Can you work these out from the model? Positions are in its coordinate system, mm. Face numbers are marked on the shaded views. Coordinates: 2 decimals unless noted, no trailing zeros. Order: outer loops, then holes, each group sorted by start corner. A loop starts at its lowest first (then second) coordinate and runs counter-clockwise, first axis right, second up. Notation, with made-up numbers: (34.5, -24) - (52.5, -24) arc R27 ccw to (52.5, -4) - close; hole circle Ø10 at (67.5, 54). An arc over 180 degrees is marked (long way). Use a Markdown table: item, result. Add a question column.
(1) I want a section at B-B (y = 2.05). List the corners of the cut face in (x, z) for me.
(2) I want a section at C-C (z = -0.5). List the corners of the cut face in (x, y) for me.
(3) If I drill on L1, parallel to Z at x = 22.25, y = 1.3; L2, parallel to Y at x = 6, z = 0.25; L3, parallel to Y at x = 10, z = 1, over which ranges is the centre line in solid material (lowest first)? Write a range as [from, to].
(4) I want a section at A-A (z = 2). List the corners of the cut face in (x, y) for me, and give its area (3 significant figures).
(5) We'd pull the mould along Z, two halves only. Please class the marked faces 1, 2 and 3: pulls with the +Z half, pulls with the -Z half, needs draft (parallel to the pull), parting line crosses it, or undercut.
(6) I want a section at D-D (z = 5.75). List the corners of the cut face in (x, y) for me, and give its area (3 significant figures).
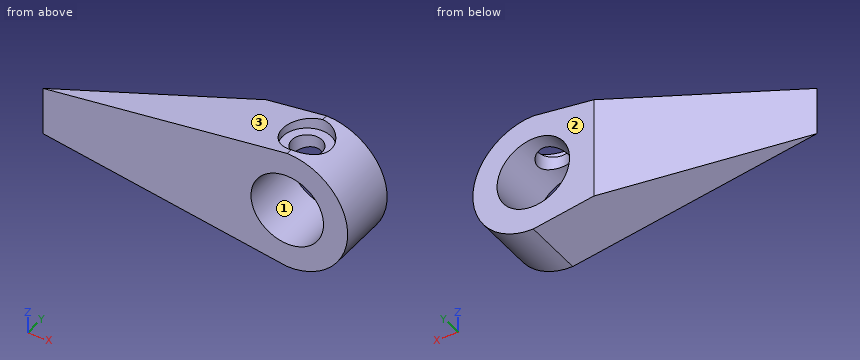
```python
from build123d import *

# Parameters (mm, degrees)
BOSS_EXTRUDE4_DEPTH     = 4
BOSS_EXTRUDE6_DEPTH     = 5
CUT_EXTRUDE3_REACH      = 28.627
CUT_EXTRUDE2_REACH      = 28.627
SKETCH9_R               = 3
CUT_EXTRUDE4_REACH      = 29.568
CUT_EXTRUDE4_END_RADIUS = 3
SKETCH12_R              = 1.25
SKETCH13_R              = 2
CUT_EXTRUDE5_DEPTH      = 1


with BuildPart() as part:
    # Sketch1 → Boss-Extrude4 (new body)
    with BuildSketch(Plane.XY):
        Polygon((0, 0), (15.198684154, 5), (15.198684154, 0), align=None)
    extrude(amount=BOSS_EXTRUDE4_DEPTH)

    # Sketch7 → Boss-Extrude6 (add)
    with BuildSketch(Plane(origin=(0, 0, 0), x_dir=(1, 0, 0), z_dir=(0, 1, 0))):
        with BuildLine():
            Line((20.198684154, 3), (0, 0))
            Line((0, 0), (15.198684154, 0))
            Line((15.198684154, 0), (15.198684154, -4))
            Line((15.198684154, -4), (0, -4))
            Line((0, -4), (20.198684154, -7))
            ThreePointArc((20.198684154, -7), (25.198684154, -2), (20.198684154, 3))
        make_face()
    extrude(amount=BOSS_EXTRUDE6_DEPTH)

    # Sketch10 → Cut-Extrude3 (cut, up to next)
    with BuildSketch(Plane.XY, mode=Mode.PRIVATE) as cut_extrude3_sk1:
        Polygon((0, 0), (0, 5), (15.198684154, 5), align=None)
    cut_extrude3_tool1 = extrude(cut_extrude3_sk1.sketch, amount=-CUT_EXTRUDE3_REACH, mode=Mode.PRIVATE) & part.part
    cut_extrude3 = cut_extrude3_tool1.solids().sort_by_distance((5.066228, 3.333333, 0))[0]
    add(cut_extrude3, mode=Mode.SUBTRACT)

    # Sketch9 → Cut-Extrude2 (cut, up to next)
    with BuildSketch(Plane(origin=(0, 5, 0), x_dir=(1, 0, 0), z_dir=(0, 1, 0)), mode=Mode.PRIVATE) as cut_extrude2_sk1:
        with Locations(Location((20.198684154, -2, 0), (0, 0, 270))):
            Circle(SKETCH9_R)
    cut_extrude2_tool1 = extrude(cut_extrude2_sk1.sketch, amount=-CUT_EXTRUDE2_REACH, mode=Mode.PRIVATE) & part.part
    add(cut_extrude2_tool1.solids().sort_by_distance((20.198684, 5, 2))[0], mode=Mode.SUBTRACT)

    # Mirror1: Cut-Extrude3 across plane
    add(cut_extrude3.mirror(Plane.XY.offset(2)), mode=Mode.SUBTRACT)

    # Cut-Extrude4: up to this cylinder (the profile starts outside it)
    cut_extrude4_end = Plane(origin=(20.198684154, 2.5, 2), z_dir=(0, 1, 0)) * Cylinder(CUT_EXTRUDE4_END_RADIUS, 66.136, mode=Mode.PRIVATE)
    # Sketch12 → Cut-Extrude4 (cut, up to the surface)
    with BuildSketch(Plane.XY.offset(7), mode=Mode.PRIVATE) as cut_extrude4_sk1:
        with Locations(Location((20.198684154, 2.5, 0), (0, 0, 270))):
            Circle(SKETCH12_R)
    cut_extrude4_tool1 = extrude(cut_extrude4_sk1.sketch, amount=-CUT_EXTRUDE4_REACH, mode=Mode.PRIVATE) - cut_extrude4_end
    add(cut_extrude4_tool1.solids().sort_by_distance((20.198684, 2.5, 7))[0], mode=Mode.SUBTRACT)

    # Sketch13 → Cut-Extrude5 (cut)
    with BuildSketch(Plane.XY.offset(7)):
        with Locations((20.198684154, 2.5)):
            Circle(SKETCH13_R)
    extrude(amount=-CUT_EXTRUDE5_DEPTH, mode=Mode.SUBTRACT)


solid = part.part
```
Answers follow:
| question | item | result |
|---|---|---|
| 1 | outline | (6.23, -0.93) - (20.2, -3) arc R5 ccw to (22.15, 6.6) - (22.15, 6) - (21.36, 6) - (21.36, 4.76) arc R3 cw (long way) to (19.03, 4.76) - (19.03, 6) - (18.25, 6) - (18.25, 6.71) - (6.23, 4.93) - close |
| 2 | outline | (3.37, 0) - (18.54, 0) - (18.54, 5) - (15.2, 5) - (3.37, 1.11) - close; (21.86, 0) - (24.53, 0) - (24.53, 5) - (21.86, 5) - close |
| 3 | L1 | z = [-2.56, -0.19], [4.19, 6.56] |
| 3 | L2 | y = [0, 1.97] |
| 3 | L3 | y = [0, 3.29] |
| 4 | outline | (0, 0) - (17.2, 0) - (17.2, 5) - (15.2, 5) - close; (23.2, 0) - (25.2, 0) - (25.2, 5) - (23.2, 5) - close |
| 4 | area | 58.0 mm² |
| 5 | face 1 | undercut |
| 5 | face 2 | needs draft |
| 5 | face 3 | pulls with the +Z half |
| 6 | outline | (11.78, 0) - (23.51, 0) - (23.51, 5) - (15.2, 5) - (11.78, 3.88) - close; hole circle Ø2.5 at (20.2, 2.5) |
| 6 | area | 51.8 mm² |
